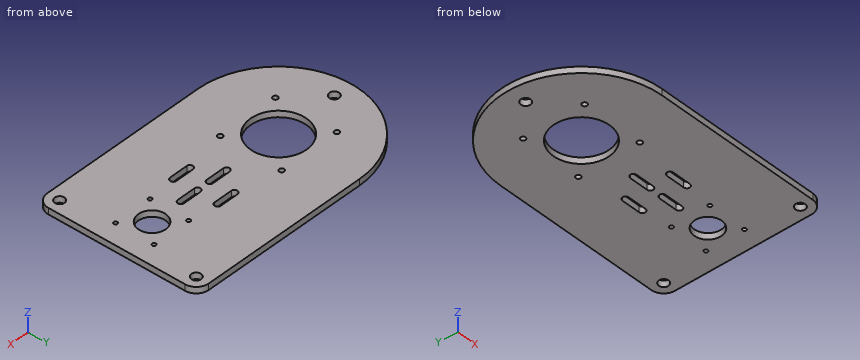
from build123d import *

# Parameters (mm, degrees)
SKETCH1_R           = 3.9
SKETCH1_R_2         = 22.5
SKETCH1_R_3         = 1.975
SKETCH1_R_4         = 11
SKETCH1_R_5         = 1.5
BOSS_EXTRUDE3_DEPTH = 5


with BuildPart() as part:
    # Sketch1 → Boss-Extrude3 (new body)
    with BuildSketch(Plane.XY):
        with BuildLine():
            Line((-40, -65), (95, -65))
            ThreePointArc((95, -65), (102.071067812, -62.071067812), (105, -55))
            Line((105, -55), (105, 55))
            ThreePointArc((105, 55), (102.071067812, 62.071067812), (95, 65))
            Line((95, 65), (-40, 65))
            ThreePointArc((-40, 65), (-105, 0), (-40, -65))
        make_face()
        with Locations((95, 55)):
            Circle(SKETCH1_R, mode=Mode.SUBTRACT)
        with Locations((95, -55)):
            Circle(SKETCH1_R, mode=Mode.SUBTRACT)
        with Locations((-90, 0)):
            Circle(SKETCH1_R, mode=Mode.SUBTRACT)
        with Locations((-40, 0)):
            Circle(SKETCH1_R_2, mode=Mode.SUBTRACT)
        with Locations((-64.75, 24.75)):
            Circle(SKETCH1_R_3, mode=Mode.SUBTRACT)
        with Locations((-15.25, 24.75)):
            Circle(SKETCH1_R_3, mode=Mode.SUBTRACT)
        with Locations((-15.25, -24.75)):
            Circle(SKETCH1_R_3, mode=Mode.SUBTRACT)
        with Locations((-64.75, -24.75)):
            Circle(SKETCH1_R_3, mode=Mode.SUBTRACT)
        with Locations((73.4, 0)):
            Circle(SKETCH1_R_4, mode=Mode.SUBTRACT)
        with Locations((57.9, 15.5)):
            Circle(SKETCH1_R_5, mode=Mode.SUBTRACT)
        with Locations((88.9, 15.5)):
            Circle(SKETCH1_R_5, mode=Mode.SUBTRACT)
        with Locations((88.9, -15.5)):
            Circle(SKETCH1_R_5, mode=Mode.SUBTRACT)
        with Locations((57.9, -15.5)):
            Circle(SKETCH1_R_5, mode=Mode.SUBTRACT)
        with BuildLine():
            Line((32.5, 2.4), (47.5, 2.4))
            ThreePointArc((47.5, 2.4), (50, -0.1), (47.5, -2.6))
            Line((47.5, -2.6), (32.5, -2.6))
            ThreePointArc((32.5, -2.6), (30, -0.1), (32.5, 2.4))
        make_face(mode=Mode.SUBTRACT)
        with BuildLine():
            Line((19.5, 20.4), (34.5, 20.4))
            ThreePointArc((34.5, 20.4), (37, 17.9), (34.5, 15.4))
            Line((34.5, 15.4), (19.5, 15.4))
            ThreePointArc((19.5, 15.4), (17, 17.9), (19.5, 20.4))
        make_face(mode=Mode.SUBTRACT)
        with BuildLine():
            Line((21.5, 2.4), (6.5, 2.4))
            ThreePointArc((6.5, 2.4), (4, -0.1), (6.5, -2.6))
            Line((6.5, -2.6), (21.5, -2.6))
            ThreePointArc((21.5, -2.6), (24, -0.1), (21.5, 2.4))
        make_face(mode=Mode.SUBTRACT)
        with BuildLine():
            Line((34.5, -15.4), (19.5, -15.4))
            ThreePointArc((19.5, -15.4), (17, -17.9), (19.5, -20.4))
            Line((19.5, -20.4), (34.5, -20.4))
            ThreePointArc((34.5, -20.4), (37, -17.9), (34.5, -15.4))
        make_face(mode=Mode.SUBTRACT)
    extrude(amount=BOSS_EXTRUDE3_DEPTH)


solid = part.part
The listing builds one solid part. Answer for the finished solid, in the listing's coordinates (mm). Give positions to 0.01 mm unless a question says otherwise; leave off trailing zeros. Loops run counter-clockwise (first coordinate to the right, second up) from the corner with the lowest first, then second, coordinate; pieces in that order, holes last.
Item 1: A cutting plane is placed at D-D (y = 49). Give the vertices of the cut face in (x, z).
Derived:
outline: (-82.71, 0) - (105, 0) - (105, 5) - (-82.71, 5) - close
Item 2: A cutting plane is placed at C-C (x = 66.5). Give the vertices of the cut face in (y, z), then the cut area to 3 significant figures.
Derived:
outline: (-65, 0) - (-8.57, 0) - (-8.57, 5) - (-65, 5) - close; (8.57, 0) - (65, 0) - (65, 5) - (8.57, 5) - close
area: 564 mm2
Item 3: This flat-tipped pin is pushed along its axis until it touches: pin 1 Ø1 at (y, z) = (2.5, 2.5) entering from -X. Where does it stop, or does it pass through?
Derived:
pin 1: stops at x = -104.97
Item 4: A cutting plane is placed at B-B (z = 2.4). Give the number of separate pieces and of enclosed holes in the cut face, then the cut area to 3 significant figures.
Derived:
separate pieces: 1
enclosed holes: 17
area: 22,900 mm2
Item 5: Find the intervals of material crossed by line 1 along Y through (x, z) = (57.9, 3.05); line 2 along Y through (x, z) = (95, 3.7); line 3 along X through (y, z) = (8, 0.7), in increasing order.
Derived:
line 1: y = -65 to -17, -14 to 14, 17 to 65
line 2: y = -65 to -58.9, -51.1 to 51.1, 58.9 to 65
line 3: x = -104.51 to -61.03, -18.97 to 65.85, 80.95 to 105
Item 6: A cutting plane is placed at A-A (x = 9.5). Give the vertices of the cut face in (y, z).
Derived:
outline: (-65, 0) - (-2.6, 0) - (-2.6, 5) - (-65, 5) - close; (2.4, 0) - (65, 0) - (65, 5) - (2.4, 5) - close
